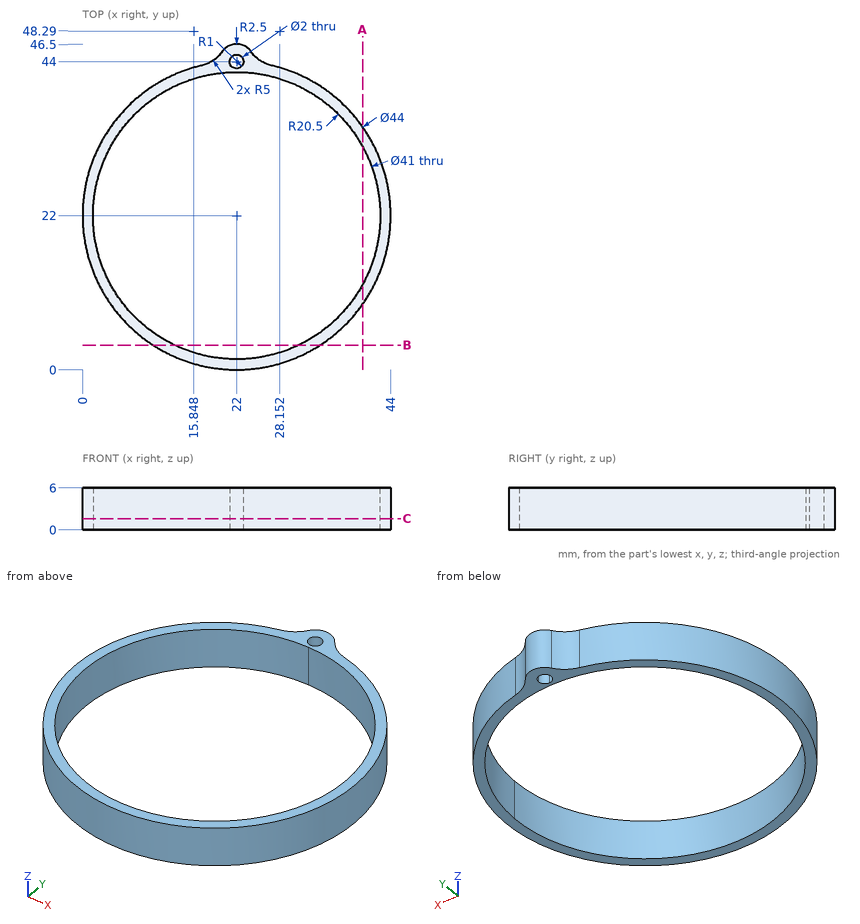
Verification items for this drawing (mm, ordinates from the low corner). Coordinates: 2 decimals unless noted, no trailing zeros. Loops run counter-clockwise (first coordinate to the right, second up) from the corner with the lowest first, then second, coordinate; pieces in that order, holes last.
Item 1: Sectioned sample at B-B, the plane y = 3.5. Record the boundary of the cut face in (x, z).
Item 2: Thickness scan on line 1 (Y direction, x = 22, z = 2.7); line 2 (X direction, y = 22, z = 1.4); line 3 (X direction, y = 12, z = 2) (1 decimal). Record the ranges inside material, lowest first.
Item 3: Sectioned sample at A-A, the plane x = 40. Record the boundary of the cut face in (y, z).
Item 4: Go/stop test with flat-tipped pins: pin 1 Ø1 at (x, z) = (26, 4) entering from +Y; pin 2 Ø1 at (y, z) = (7.5, 5) entering from -X. Record where each tip stops, or that it passes through.
Item 5: Sectioned sample at C-C, the plane z = 1.6. Record the boundary of the cut face in (x, y), then the cut area to 3 significant figures.
Check result:
1. outline: (10.09, 0) - (13.17, 0) - (13.17, 6) - (10.09, 6) - close; (30.83, 0) - (33.91, 0) - (33.91, 6) - (30.83, 6) - close
2. line 1: y = 0 to 1.5, 42.5 to 43, 45 to 46.5
2. line 2: x = 0 to 1.5, 42.5 to 44
2. line 3: x = 2.4 to 4.1, 39.9 to 41.6
3. outline: (9.35, 0) - (12.19, 0) - (12.19, 6) - (9.35, 6) - close; (31.81, 0) - (34.65, 0) - (34.65, 6) - (31.81, 6) - close
4. pin 1: stops at y = 44.05
4. pin 2: stops at x = 5.03
5. outline: (16.99, 43.42) arc R22 ccw (long way) to (27.01, 43.42) arc R5 cw to (24.05, 45.43) arc R2.5 ccw to (19.95, 45.43) arc R5 cw to start; hole circle Ø41 at (22, 22); hole circle Ø2 at (22, 44)
5. area: 209 mm2
